```python
from build123d import *

# Parameters (mm, degrees)
SKETCH1_R           = 3.135927073
SKETCH1_R_2         = 2.01
BOSS_EXTRUDE1_DEPTH = 5
CUT_EXTRUDE4_DEPTH  = 4
SKETCH4_R           = 0.99
BOSS_EXTRUDE3_DEPTH = 10


with BuildPart() as part:
    # Sketch1 → Boss-Extrude1 (new body)
    # profile 1 of 4: a face of its own
    with BuildSketch(Plane(origin=(0, 0, 0), x_dir=(1, 0, 0), z_dir=(0, 1, 0))):
        with Locations(Location((0, 0, 0), (0, 0, 270))):
            Circle(SKETCH1_R)
        Circle(SKETCH1_R_2, mode=Mode.SUBTRACT)
    # profile 2 of 4: a face of its own
    with BuildSketch(Plane(origin=(0, 0, 0), x_dir=(1, 0, 0), z_dir=(0, 1, 0))):
        with BuildLine():
            Line((1.48610851, 1.353359337), (-1.48610851, 1.353359337))
            ThreePointArc((-1.48610851, 1.353359337), (-2.009995593, 0.004208893), (-1.491763272, -1.347123729))
            Line((-1.491763272, -1.347123729), (1.491763272, -1.347123729))
            ThreePointArc((1.491763272, -1.347123729), (1.875972305, -0.721684081), (2.01, 0))
            ThreePointArc((2.01, 0), (1.874457002, 0.725610741), (1.48610851, 1.353359337))
        make_face()
    # profile 3 of 4: a face of its own
    with BuildSketch(Plane(origin=(0, 0, 0), x_dir=(1, 0, 0), z_dir=(0, 1, 0))):
        with BuildLine():
            ThreePointArc((1.48610851, 1.353359337), (0, 2.01), (-1.48610851, 1.353359337))
            Line((-1.48610851, 1.353359337), (1.48610851, 1.353359337))
        make_face()
    # profile 4 of 4: a face of its own
    with BuildSketch(Plane(origin=(0, 0, 0), x_dir=(1, 0, 0), z_dir=(0, 1, 0))):
        with BuildLine():
            Line((1.491763272, -1.347123729), (-1.491763272, -1.347123729))
            ThreePointArc((-1.491763272, -1.347123729), (0, -2.01), (1.491763272, -1.347123729))
        make_face()
    extrude(amount=BOSS_EXTRUDE1_DEPTH)

    # Sketch2 → Cut-Extrude4 (cut)
    with BuildSketch(Plane(origin=(0, 0, 0), x_dir=(1, 0, 0), z_dir=(0, 1, 0))):
        with BuildLine():
            Line((-1.995763722, -1.58727035), (1.995763722, -1.58727035))
            ThreePointArc((1.995763722, -1.58727035), (2.407456904, -0.840625514), (2.55, 0))
            ThreePointArc((2.55, 0), (2.407456904, 0.840625514), (1.995763722, 1.58727035))
            Line((1.995763722, 1.58727035), (-1.995763722, 1.58727035))
            ThreePointArc((-1.995763722, 1.58727035), (-2.55, 0), (-1.995763722, -1.58727035))
        make_face()
    extrude(amount=CUT_EXTRUDE4_DEPTH, mode=Mode.SUBTRACT)

    # Sketch4 → Boss-Extrude3 (add)
    with BuildSketch(Plane(origin=(0, 5, 0), x_dir=(1, 0, 0), z_dir=(0, 1, 0))):
        with Locations(Location((0, 0, 0), (0, 0, 270))):
            Circle(SKETCH4_R)
    extrude(amount=BOSS_EXTRUDE3_DEPTH)


solid = part.part
```
Geometry: final body of the model. Coordinates: model frame, mm. A direction names the side the tool comes from. Coordinates: 2 decimals unless noted, no trailing zeros. Order: outer loops, then holes, each group sorted by start corner. A loop starts at its lowest first (then second) coordinate and runs counter-clockwise, first axis right, second up. Notation, with made-up numbers: (51, 12) -> (81, 12) arc R19 cw to (81, 41) -> close; hole circle Ø1 at (5, 72). An arc over 180 degrees is marked (long way). Use CSV: the item, a comma, the result in double quotes.
1) Section C-C on z = -1.25. Output: boundary loops of the cut face in (x, y).
Findings:
outline,"(-2.88, 0) -> (-2.22, 0) -> (-2.22, 4) -> (2.22, 4) -> (2.22, 0) -> (2.88, 0) -> (2.88, 5) -> (-2.88, 5) -> close"
2) Mould query, pull axis Z, two halves, no side actions, for faces 1 (the flat face through (0, 2, -1.587)), 2 (the cylindrical face through (-0.966, 9.93, -0.215)), 3 (the flat face through (0, 15, 0)), 4 (the cylindrical face through (-2.55, 1.97, -0.02)). Classes: +Z half, -Z half, draft (parallel to the pull), parting line (faces both ways), or undercut.
Findings:
face 1,"undercut"
face 2,"parting line"
face 3,"draft"
face 4,"undercut"
3) Section A-A on y = 2.25. Output: boundary loops of the cut face in (x, z), then the cut area to 3 significant figures.
Findings:
outline,"circle Ø6.27 at (0, 0); hole (-2, -1.59) -> (2, -1.59) arc R2.55 ccw to (2, 1.59) -> (-2, 1.59) arc R2.55 ccw to start"
area,"15.8 mm^2"
4) Access query for faces 5 (the flat face through (1, 5, -1)), 6 (the cylindrical face through (-2.78, 2.46, 1.45)), 7 (the flat face through (0, 4, 0)). Directions: +Z, -Z, +X, -X, +Y, -Y. A direction counts if a zero-diameter tool reaches every point of the face in a straight line with its end or side. Return the directions, or none.
Findings:
face 5,"+Y"
face 6,"+Y, -Y"
face 7,"-Y"
5) Line query: line 1 (Y direction, x = 0.75, z = 1.5); line 2 (X direction, y = 3.5, z = 1.25); line 3 (Y direction, x = -2.5, z = -0.75). Output: solid intervals per line, ascending.
Findings:
line 1,"y = 4 to 5"
line 2,"x = -2.88 to -2.22, 2.22 to 2.88"
line 3,"y = 0 to 5"
6) Section B-B on x = 0. Output: boundary loops of the cut face in (y, z).
Findings:
outline,"(0, -3.14) -> (5, -3.14) -> (5, -0.99) -> (15, -0.99) -> (15, 0.99) -> (5, 0.99) -> (5, 3.14) -> (0, 3.14) -> (0, 1.59) -> (4, 1.59) -> (4, -1.59) -> (0, -1.59) -> close"
7) Section D-D on y = 13.5. Output: boundary loops of the cut face in (x, z), then the cut area to 3 significant figures.
Findings:
outline,"circle Ø1.98 at (0, 0)"
area,"3.08 mm^2"
